from build123d import *

# Parameters (mm, degrees)
F0_W     = 8
F0_H     = 26
F1_DEPTH = 12.5
F3_DEPTH = 4
F5_DEPTH = 25


with BuildPart() as f1:
    # F0 (on Right) → F1 (new body, symmetric)
    with BuildSketch(Plane.YZ):
        with Locations((4, 13)):
            Rectangle(F0_W, F0_H)
        with BuildLine():
            ThreePointArc((8, 26), (4, 30), (0, 26))
            Line((0, 26), (8, 26))
        make_face()
    extrude(amount=F1_DEPTH, both=True)

    # F2 (on Right) → F3 (join, symmetric)
    with BuildSketch(Plane.YZ):
        Polygon((8, 24), (8, 0), (22, 0), (22, 2), (10, 24), align=None)
    extrude(amount=F3_DEPTH, both=True)

    # F4 (on Front) → F5 (cut)
    with BuildSketch(Plane.XZ):
        with BuildLine():
            Line((-10.5, 30), (-12.5, 30))
            Line((-12.5, 30), (-12.5, 28))
            ThreePointArc((-12.5, 28), (-11.914214, 29.414214), (-10.5, 30))
        make_face()
        with BuildLine():
            ThreePointArc((10.5, 30), (11.914214, 29.414214), (12.5, 28))
            Line((12.5, 28), (12.5, 30))
            Line((12.5, 30), (10.5, 30))
        make_face()
    extrude(amount=-F5_DEPTH, mode=Mode.SUBTRACT)


solid = f1.part
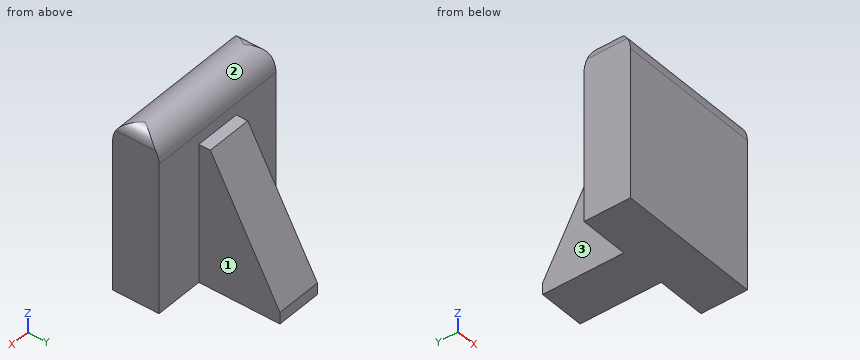
Read the model definition and answer for the solid it produces. Units are mm, in the model's axes. Face numbers are marked on the shaded views. A direction names the side the tool comes from. Give positions to 0.01 mm unless a question says otherwise; leave off trailing zeros. Loops run counter-clockwise (first coordinate to the right, second up) from the corner with the lowest first, then second, coordinate; pieces in that order, holes last. Notation, with made-up numbers: (-35, -21.5) - (-29, -21.5) arc R20 cw to (-29, 1.5) - close; hole circle Ø1 at (68, -5.75). An arc over 180 degrees is marked (long way). Answer as CSV lines item,"result". Start each with the question number.
1) Find section B-B (x = -9.25). Write down the section's boundary in (y, z), then the cut area to 3 significant figures.
2) Find section D-D (z = 10). Write down the section's boundary in (x, y).
3) Find section A-A (z = 19.5). Write down the section's boundary in (x, y), then the cut area to 3 significant figures.
4) Which of the six approach directions +Z, -Z, +X, -X, +Y, -Y give full straight-line access (tool end or side, diameter ignored) to the marked faces 1, 2 and 3?
5) Find section C-C (y = 7). Write down the section's boundary in (x, z), then the cut area to 3 significant figures.
6) Straight lines are drawn through the part: L1, parallel to Y at x = -6.25, z = 14; L2, parallel to X at y = 9.75, z = 18.5; L3, parallel to Z at x = 2, y = 17. For each, find the intervals that lie inside material, in ascending order. Write a range as from..to.
7) Each of these flat-tipped pins is pushed along its axis until it touches: pin 1 Ø3 at (x, y) = (2.5, 4.5) entering from +Z; pin 2 Ø7.5 at (x, z) = (0.5, 15) entering from +Y; pin 3 Ø3 at (x, y) = (-6, 8.5) entering from +Z; pin 4 Ø4 at (x, y) = (-6.5, 19) entering from -Z. Where does it stop, or does it pass through?
Findings below:
1,outline,"(0, 0) - (8, 0) - (8, 26) arc R4 ccw to (0, 26) - close"
1,area,"233 mm^2"
2,outline,"(-12.5, 0) - (12.5, 0) - (12.5, 8) - (4, 8) - (4, 17.64) - (-4, 17.64) - (-4, 8) - (-12.5, 8) - close"
3,outline,"(-12.5, 0) - (12.5, 0) - (12.5, 8) - (4, 8) - (4, 12.45) - (-4, 12.45) - (-4, 8) - (-12.5, 8) - close"
3,area,"236 mm^2"
4,face 1,"+Z, -Z, +X, +Y"
4,face 2,"+Z, +X, -X"
4,face 3,"+Z, -Z, -X, +Y"
5,outline,"(-12.5, 0) - (12.5, 0) - (12.5, 28) arc R2 ccw to (12.39, 28.65) - (-12.39, 28.65) arc R2 ccw to (-12.5, 28) - close"
5,area,"716 mm^2"
6,L1,"0..8"
6,L2,"-4..4"
6,L3,"0..11.17"
7,pin 1,"z = 30"
7,pin 2,"y = 16.95"
7,pin 3,"z = 28.65"
7,pin 4,"through"
